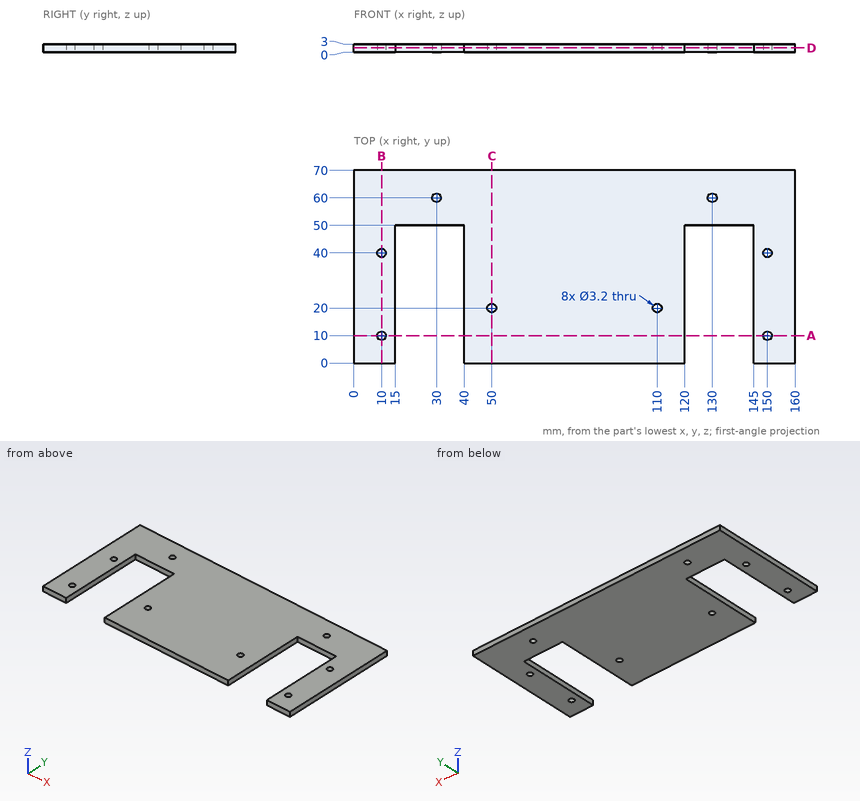
Geometry check sheet. Reference: drawing and pictorial views, mm from the part's lowest x, y, z. Round coordinates to 2 decimals unless told otherwise and drop trailing zeros. Order: outer loops, then holes, each group sorted by start corner. A loop starts at its lowest first (then second) coordinate and runs counter-clockwise, first axis right, second up. Notation, with made-up numbers: M -30,-2.5 L 19,-2.5 A20 ccw 19,35.5 Z; hole C 38,-25 d5. An arc over 180 degrees is marked long. Answer in a Markdown table with one row per item.
(1) Sectioned sample at A-A, the plane y = 10. Record the cut outline in (x, z), and give its area (3 significant figures).
Responses:
| item | result |
|---|---|
| outline | M 0,0 L 8.4,0 L 8.4,3 L 0,3 Z; M 11.6,0 L 15,0 L 15,3 L 11.6,3 Z; M 40,0 L 120,0 L 120,3 L 40,3 Z; M 145,0 L 148.4,0 L 148.4,3 L 145,3 Z; M 151.6,0 L 160,0 L 160,3 L 151.6,3 Z |
| area | 311 mm² |
(2) Scan lines: probe 1 along X at (y, z) = (40, 2.75); probe 2 along X at (y, z) = (60, 1.4); probe 3 along X at (y, z) = (32, 0.95). Record each from-to range of solid material in increasing order. Write a range as from..to.
Responses:
| item | result |
|---|---|
| probe 1 | x = 0..8.4, 11.6..15, 40..120, 145..148.4, 151.6..160 |
| probe 2 | x = 0..28.4, 31.6..128.4, 131.6..160 |
| probe 3 | x = 0..15, 40..120, 145..160 |
(3) Go/stop test with flat-tipped pins: P1, Ø4, axis at x = 50, y = 20, coming from the -Z side; P2, Ø3, axis at x = 110, y = 20, coming from the +Z side; P3, Ø1.5, axis at x = 23, z = 1.5, coming from the -Y side. Record where each tip stops, or that it passes through.
Responses:
| item | result |
|---|---|
| P1 | stops at z = 0 |
| P2 | passes through |
| P3 | stops at y = 50 |
(4) Sectioned sample at D-D, the plane z = 1.55. State how many separate pieces and enclosed holes the cut face has, and give its area (3 significant figures).
Responses:
| item | result |
|---|---|
| separate pieces | 1 |
| enclosed holes | 8 |
| area | 8,640 mm² |
(5) Sectioned sample at B-B, the plane x = 10. Record the cut outline in (y, z), and give its area (3 significant figures).
Responses:
| item | result |
|---|---|
| outline | M 0,0 L 8.4,0 L 8.4,3 L 0,3 Z; M 11.6,0 L 38.4,0 L 38.4,3 L 11.6,3 Z; M 41.6,0 L 70,0 L 70,3 L 41.6,3 Z |
| area | 191 mm² |
(6) Sectioned sample at C-C, the plane x = 50. Record the cut outline in (y, z).
Responses:
| item | result |
|---|---|
| outline | M 0,0 L 18.4,0 L 18.4,3 L 0,3 Z; M 21.6,0 L 70,0 L 70,3 L 21.6,3 Z |
